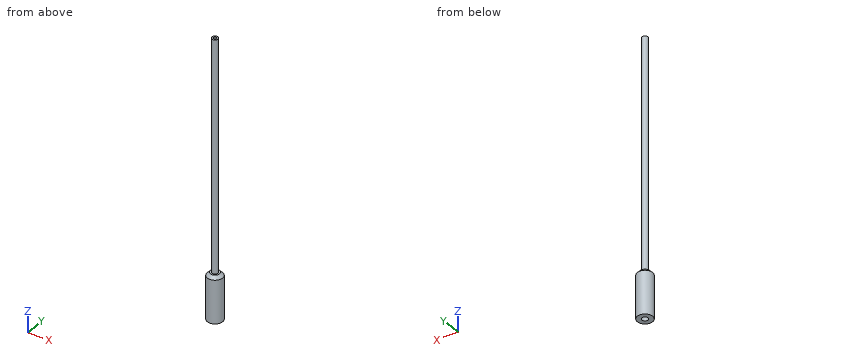
from build123d import *

# Parameters (mm, degrees)
F0_R     = 12.7
F0_R_2   = 5.08
F0_R_3   = 2.54
F1_DEPTH = 76.2
F2_DEPTH = 58.42
F3_START = 71.628
F3_DEPTH = 385.572
F4_SIZE  = 5.08


with BuildPart() as f1:
    # F0 (on Top) → F1 (new body)
    with BuildSketch(Plane.XY):
        Circle(F0_R)
        Circle(F0_R_2, mode=Mode.SUBTRACT)
        Circle(F0_R_2)
        Circle(F0_R_3, mode=Mode.SUBTRACT)
        Circle(F0_R_3)
    extrude(amount=F1_DEPTH)

    # F0 (on Top) → F2 (cut)
    with BuildSketch(Plane.XY):
        Circle(F0_R_2)
        Circle(F0_R_3, mode=Mode.SUBTRACT)
        Circle(F0_R_3)
    extrude(amount=F2_DEPTH, mode=Mode.SUBTRACT)

    # F0 (on Top) → F3 (join)
    with BuildSketch(Plane.XY.offset(F3_START)):
        Circle(F0_R_2)
        Circle(F0_R_3, mode=Mode.SUBTRACT)
    extrude(amount=F3_DEPTH)

    # F4
    f4_edges = [f1.edges().sort_by_distance(p)[0] for p in [
        (-12.7, 0, 76.2),
    ]]
    chamfer(f4_edges, length=F4_SIZE)


solid = f1.part
The listing builds one solid part. Answer for the finished solid, in the listing's coordinates (mm). Give positions to 0.01 mm unless a question says otherwise; leave off trailing zeros. Write each loop counter-clockwise with the first axis right and the second up, starting at its lowest first coordinate (ties: lowest second). Pieces come first, ordered by that corner, then holes. Notation, with made-up numbers: (8, -18) -> (67, -18) arc R12 cw to (67, -6) -> close; hole circle Ø7 at (6.25, 87.25). An arc over 180 degrees is marked (long way). One line per question, with ' | ' between items. Start each with the question number.
1. Given pin 1 Ø3 at (y, z) = (-8.5, 406) entering from +X; pin 2 Ø10 at (x, y) = (-3.5, 6.5) entering from -Z; pin 3 Ø4 at (x, z) = (1, 338) entering from -Y; pin 4 Ø3 at (y, z) = (2.5, 90.5) entering from -X, each flat-ended and moving along its own axis, determine where each tip first touches the part or whether it passes through.
2. Section A-A (z = 293.5) is taken. Determine the outline of the cut face in (x, y), plus the area to 3 significant figures.
3. Find the intervals of material crossed by probe 1 along Y at (x, z) = (0, 180.5); probe 2 along Z at (x, y) = (4.75, -6), in increasing order.
Response values:
1) pin 1: through | pin 2: z = 0 | pin 3: y = -5.08 | pin 4: x = -4.98
2) outline: circle Ø10.16 at (0, 0); hole circle Ø5.08 at (0, 0) | area: 60.8 mm2
3) probe 1: -5.08 to -2.54, 2.54 to 5.08 | probe 2: 0 to 76.17
